For this review, take the finished solid that the model builds, in its own axes (mm). Coordinates: 2 decimals unless noted, no trailing zeros. Loops run counter-clockwise (first coordinate to the right, second up) from the corner with the lowest first, then second, coordinate; pieces in that order, holes last. Notation, with made-up numbers: (2.25, 79.25) - (44.25, 79.25) arc R36 cw to (44.25, 113.25) - close; hole circle Ø3 at (-19, 56). An arc over 180 degrees is marked (long way). Answer as a JSON object with one key per item and string values. Group by question number.
Item 1: We need section B-B (y = -4.5). Give the boundary of the cut face in (x, z).
Item 2: We need section C-C (z = 0.3). State how many separate pieces and enclosed holes the cut face has, then the cut area to 3 significant figures.
Item 3: We need section D-D (x = 22). Give the boundary of the cut face in (y, z).
Item 4: We need section A-A (x = 29.5). Give the boundary of the cut face in (y, z).
Item 5: To check wall thickness, follow line 1 (Y direction, x = 37, z = 0.2); line 2 (X direction, y = -38, z = 0.45); line 3 (X direction, y = -20, z = 0.25). State the ranges of each line that lie inside material, in increasing order.
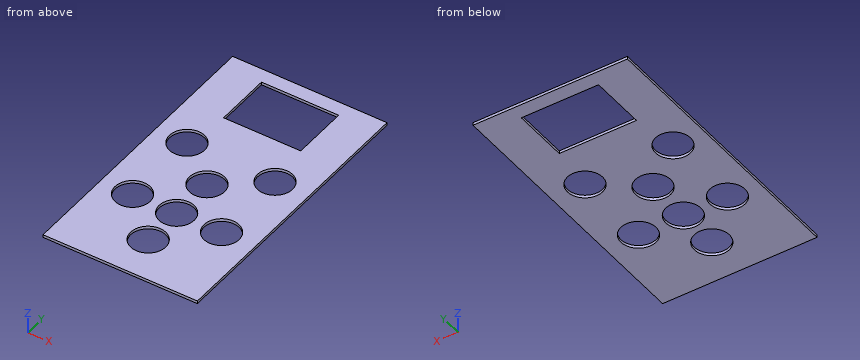
from build123d import *

# Parameters (mm, degrees)
SKETCH_1_W      = 55
SKETCH_1_H      = 100
SKETCH_1_R      = 6.25
SKETCH_1_W_2    = 27.5
SKETCH_1_H_2    = 20
EXTRUDE_1_DEPTH = 1


with BuildPart() as part:
    # 草图1 → 凸台-拉伸1 (new body)
    with BuildSketch(Plane.XY):
        with Locations((37.918181818, -46.951515152)):
            Rectangle(SKETCH_1_W, SKETCH_1_H)
        with Locations((37.418181818, -81.451515152)):
            Circle(SKETCH_1_R, mode=Mode.SUBTRACT)
        with Locations((37.418181818, -66.451515152)):
            Circle(SKETCH_1_R, mode=Mode.SUBTRACT)
        with Locations((21.718181818, -66.451515152)):
            Circle(SKETCH_1_R, mode=Mode.SUBTRACT)
        with Locations((53.418181818, -66.451515152)):
            Circle(SKETCH_1_R, mode=Mode.SUBTRACT)
        with Locations((37.418181818, -50.451515152)):
            Circle(SKETCH_1_R, mode=Mode.SUBTRACT)
        with Locations((53.418181818, -38.251515152)):
            Circle(SKETCH_1_R, mode=Mode.SUBTRACT)
        with Locations((21.718181818, -37.751515152)):
            Circle(SKETCH_1_R, mode=Mode.SUBTRACT)
        with Locations((37.918181818, -12.084434283)):
            Rectangle(SKETCH_1_W_2, SKETCH_1_H_2, mode=Mode.SUBTRACT)
    extrude(amount=EXTRUDE_1_DEPTH)


solid = part.part
Check sheet entries:
{
 "1": {"outline": "(10.42, 0) - (24.17, 0) - (24.17, 1) - (10.42, 1) - close; (51.67, 0) - (65.42, 0) - (65.42, 1) - (51.67, 1) - close"},
 "2": {"separate pieces": "1", "enclosed holes": "8", "area": "4,090 mm2"},
 "3": {"outline": "(-96.95, 0) - (-72.7, 0) - (-72.7, 1) - (-96.95, 1) - close; (-60.21, 0) - (-44, 0) - (-44, 1) - (-60.21, 1) - close; (-31.51, 0) - (3.05, 0) - (3.05, 1) - (-31.51, 1) - close"},
 "4": {"outline": "(-96.95, 0) - (-22.08, 0) - (-22.08, 1) - (-96.95, 1) - close; (-2.08, 0) - (3.05, 0) - (3.05, 1) - (-2.08, 1) - close"},
 "5": {"line 1": "y = -96.95 to -87.69, -75.22 to -72.69, -60.22 to -56.69, -44.22 to -22.08, -2.08 to 3.05", "line 2": "x = 10.42 to 15.47, 27.96 to 47.17, 59.66 to 65.42", "line 3": "x = 10.42 to 24.17, 51.67 to 65.42"}
}
